Check sheet for the drawn part. Datum: minimum x, y, z corner. Units: mm. Round coordinates to 2 decimals unless told otherwise and drop trailing zeros. Order: outer loops, then holes, each group sorted by start corner. A loop starts at its lowest first (then second) coordinate and runs counter-clockwise, first axis right, second up. Notation, with made-up numbers: (86.5, -6) -> (144.5, -6) arc R27 ccw to (144.5, 12) -> close; hole circle Ø2 at (58, -6.75). An arc over 180 degrees is marked (long way). Answer as a JSON object with one key per item and string values. Group by question number.
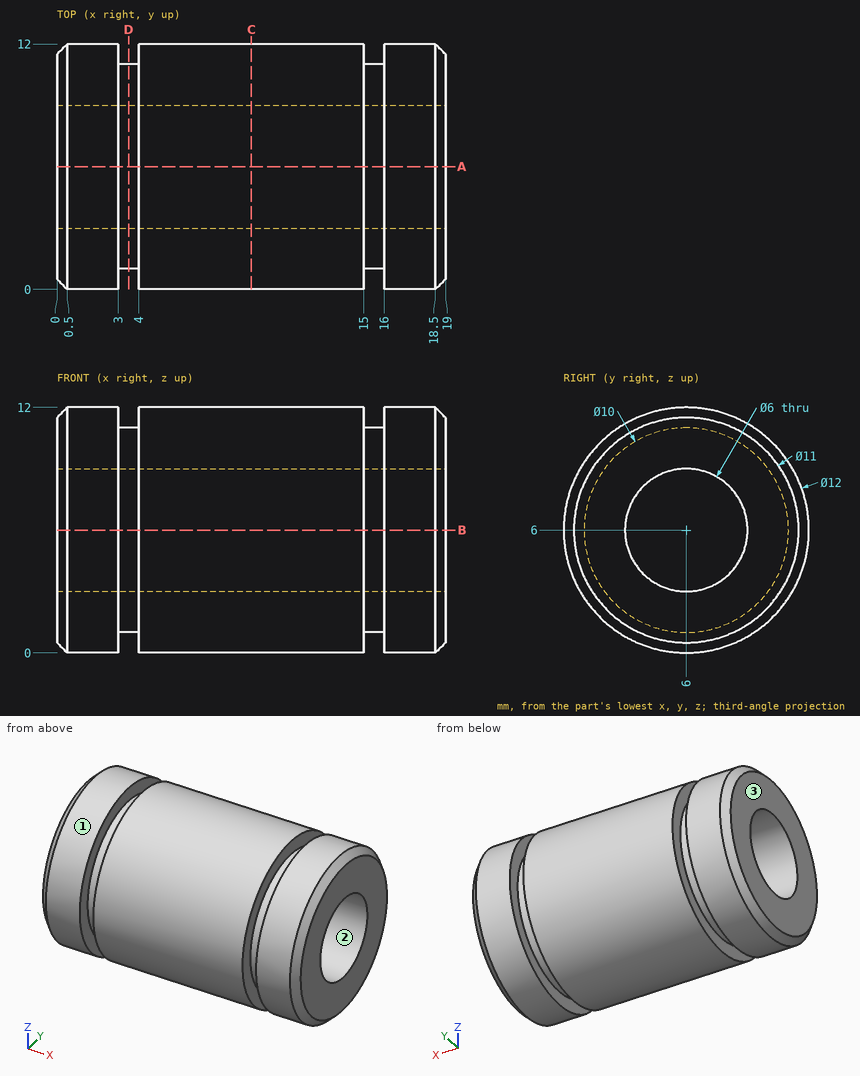
Item 1: Depth check by flat-ended pin: pin 1 Ø2 at (x, y) = (7.5, 3) entering from -Z; pin 2 Ø1.5 at (x, y) = (14.5, 1.5) entering from +Z; pin 3 Ø1.5 at (x, y) = (10.5, 5) entering from -Z. Enter the tip coordinate at first touch or a pass-through.
Item 2: Sectioned sample at D-D, the plane x = 3.5. Enter the section's corners in (y, z).
Item 3: Thickness scan on L1, parallel to X at y = 10.75, z = 3.75; L2, parallel to Y at x = 11.75, z = 6. Record the ranges inside material, lowest first.
Item 4: Mould release check, pull along Y, two halves, no side actions. Record for the marked faces 1, 2 and 3: pulls with the +Y half, pulls with the -Y half, needs draft (parallel to the pull), parting line crosses it, or undercut.
Item 5: Sectioned sample at A-A, the plane y = 6. Enter the section's corners in (x, z), then the cut area to 4 significant figures.
Item 6: Sectioned sample at C-C, the plane x = 9.5. Enter the section's corners in (y, z).
Result:
{
 "1": {"pin 1": "stops at z = 0.34", "pin 2": "stops at z = 10.68", "pin 3": "stops at z = 0.01"},
 "2": {"outline": "circle Ø10 at (6, 6); hole circle Ø6 at (6, 6)"},
 "3": {"L1": "x = 0 to 3, 4 to 15, 16 to 19", "L2": "y = 0 to 3, 9 to 12"},
 "4": {"face 1": "parting line crosses it", "face 2": "undercut", "face 3": "needs draft"},
 "5": {"outline": "(0, 0.5) -> (0.5, 0) -> (3, 0) -> (3, 1) -> (4, 1) -> (4, 0) -> (15, 0) -> (15, 1) -> (16, 1) -> (16, 0) -> (18.5, 0) -> (19, 0.5) -> (19, 3) -> (0, 3) -> close; (0, 9) -> (19, 9) -> (19, 11.5) -> (18.5, 12) -> (16, 12) -> (16, 11) -> (15, 11) -> (15, 12) -> (4, 12) -> (4, 11) -> (3, 11) -> (3, 12) -> (0.5, 12) -> (0, 11.5) -> close", "area": "109.5 mm2"},
 "6": {"outline": "circle Ø12 at (6, 6); hole circle Ø6 at (6, 6)"}
}
